Autodesk Inventor part; units mm, degrees
ref_plane "Work Plane1" through (0, 4, 0) normal (0, -1, 0) x (1, 0, 0)
ref_plane "YZ Plane" through (0, 0, 0) normal (1, 0, 0) x (0, 1, 0)
ref_plane "XZ Plane" through (0, 0, 0) normal (0, 1, 0) x (-1, 0, 0)
sketch "Sketch1" plane through (0, 0, 0) normal (0, 1, 0) x (-1, 0, 0)
  line L0 (6, 8) -> (6, -8)
  line L1 (-6, 8) -> (-6, -8)
  arc A0 (6, 8) -> (-6, 8) centre (0, 0) ccw
  arc A1 (-6, -8) -> (6, -8) centre (0, 0) ccw
  circle A2 centre (1.5, 7) radius 1.5
  line L2 (0, 0) -> (6, 0) construction
  circle A3 centre (1.5, -7) radius 1.5
  circle A4 centre (0, 0) radius 3.5
  circle A5 centre (0, 0) radius 4.3
  dimension "d0" = 10
  dimension "d1" = 10
  dimension "d3" = 12
  dimension "d4" = 3
  dimension "d5" = 7
  dimension "d6" = 1.5
  dimension "d7" = 7
  dimension "d16" = 8.6
extrude "Extrusion1" add sketch "Sketch1" along normal blind 27.8 contours L0 A1 L1 A0 | A2 | A3 | A5
ref_plane "Work Plane1" through (0, 4, 0) normal (0, -1, 0) x (1, 0, 0)
sketch "Sketch2" plane through (0, 4, 0) normal (0, -1, 0) x (1, 0, 0)
  line L0 (-6, -8) -> (-6, 8)
  arc A0 (6, 8) -> (-6, 8) centre (0, 0) ccw
  line L1 (6, 8) -> (6, -8)
  arc A1 (-6, -8) -> (6, -8) centre (0, 0) ccw
extrude "Extrusion2" cut sketch "Sketch2" against normal blind 1
pattern_linear "Rectangular Pattern1" count 9 spacing 1.8 along (0, 1, 0) of "Extrusion2"
extrude "Extrusion3" add sketch "Sketch1" along normal blind 16.7 contours A5
sketch "Sketch3" plane through (0, 16.7, 0) normal (0, 1, 0) x (1, 0, 0)
  circle A0 centre (0, 0) radius 4.3
  circle A1 centre (0, 0) radius 3
  dimension "d19" = 6
extrude "Extrusion4" add sketch "Sketch3" along normal blind 3.1
sketch "Sketch4" plane through (0, 27.8, 0) normal (0, 1, 0) x (1, 0, 0)
  circle A0 centre (0, 0) radius 5
  dimension "d22" = 10
extrude "Extrusion5" cut sketch "Sketch4" against normal blind 8
extrude "Extrusion6" cut sketch "Sketch1" along normal blind 4 contours A2 | A3
sketch "Sketch5" plane through (6, 27.8, 8) normal (1, 0, 0) x (0, 0, -1)
  circle A0 centre (1, -4) radius 1.6
  circle A1 centre (15, -4) radius 1.6
  point P0 (8, -27.8)
  dimension "d27" = 3.2
  dimension "d28" = 23.8
  dimension "d29" = 14
  dimension "d31" = 7
extrude "Extrusion7" cut sketch "Sketch5" against normal blind 12
sketch "Sketch6" plane through (6, 0, 8) normal (1, 0, 0) x (0, 0, -1)
  circle A0 centre (8, 2) radius 1.5
  line L0 (0, 0) -> (16, 0)
  point P0 (8, 0)
  point P1 (8, 0)
  dimension "d34" = 2
  dimension "d35" = 3
extrude "Extrusion8" cut sketch "Sketch6" against normal blind 4.75
properties part number "ENDER 3 RAD" material "Aluminum 6061"
Geometry check sheet. Reference: the model listing, model coordinates, mm. A direction names the side the tool comes from. Coordinates: 2 decimals unless noted, no trailing zeros. Loops run counter-clockwise (first coordinate to the right, second up) from the corner with the lowest first, then second, coordinate; pieces in that order, holes last.
Item 1: Release check for a two-part mould opening along Y. For faces 1 (the face through (-3, 18, 0)), 2 (the face through (3, 16.7, -1)), 3 (the face through (0, 4, 5)) record: released by +Y, released by -Y, zero draft, split by the parting line, or undercut.
Item 2: Sectioned sample at B-B, the plane z = 0. Count the separate pieces of the cut face and the enclosed holes in it, then the cut area to 3 significant figures.
Item 3: Sectioned sample at A-A, the plane y = 23.25. Record the boundary of the cut face in (x, z).
Item 4: Go/stop test with flat-tipped pins: pin 1 Ø7 at (x, z) = (0, 0) entering from +Y; pin 2 Ø2 at (x, y) = (-3, 12.5) entering from -Z; pin 3 Ø4 at (x, z) = (0, 0) entering from -Y. Record where each tip stops, or that it passes through.
Item 5: Thickness scan on line 1 (Z direction, x = -3.5, y = 24); line 2 (Z direction, x = 0, y = 26); line 3 (X direction, y = 3.75, z = 0). Record the ranges inside material, lowest first.
Item 6: Access from +Z, -Z, +X, -X, +Y, -Y to the whole of each face (thin tool, end or side, straight path). Record for faces 4 (the face through (-1.175, 1.972, -5.536)), 5 (the face through (4.296, 15.293, -0.189)), 6 (the face through (0, 9, 10)).
Check result:
1. face 1: zero draft
1. face 2: released by -Y
1. face 3: undercut
2. separate pieces: 3
2. enclosed holes: 0
2. area: 80.0 mm2
3. outline: (-6, -5.5) - (6, -5.5) - (6, 5.5) - (-6, 5.5) - close; (-5.26, -8.5) arc R10 ccw to (5.26, -8.5) - close; (-5.26, 8.5) - (5.26, 8.5) arc R10 ccw to start; hole circle Ø10 at (0, 0)
4. pin 1: stops at y = 19.8
4. pin 2: stops at z = -9.8
4. pin 3: passes through
5. line 1: z = -9.37 to -8.59, -5.41 to -3.57, 3.57 to 5.41, 8.59 to 9.37
5. line 2: z = -10 to -5, 5 to 10
5. line 3: x = -6 to -3.5, 3.5 to 6
6. face 4: -Y
6. face 5: none
6. face 6: +Z, +Y, -Y
